```python
from build123d import *

# Parameters (mm, degrees)
F0_R     = 3.9243
F1_DEPTH = 2.54
F2_R     = 3.4925
F3_DEPTH = 25.4
F4_W     = 2.531840682
F4_H     = 6.5099929156
F5_DEPTH = 10.16
F6_R     = 1.524
F7_DEPTH = 25.4
F8_R     = 1.14299


# Not quite as in the source:
# - a fillet or chamfer is up to 0.001 mm smaller than in the source, because OpenCascade refuses the exact size


with BuildPart() as f1:
    # F0 (on Right) → F1 (new body)
    with BuildSketch(Plane.YZ):
        Circle(F0_R)
    extrude(amount=F1_DEPTH)

    # F2 (on face) → F3 (join)
    with BuildSketch(Plane.YZ.offset(2.54)):
        Circle(F2_R)
    extrude(amount=F3_DEPTH)

    # F4 (on face) → F5 (join)
    with BuildSketch(Plane.YZ.offset(27.94)):
        Rectangle(F4_W, F4_H)
    extrude(amount=F5_DEPTH)

    # F6 (on face) → F7 (cut)
    with BuildSketch(Plane(origin=(0, 1.265920341, 0), x_dir=(-1, 0, 0), z_dir=(0, 1, 0))):
        with Locations((-33.02, 0)):
            Circle(F6_R)
    extrude(amount=-F7_DEPTH, mode=Mode.SUBTRACT)

    # F8 (radius 1.143 in the source; OpenCascade refuses exactly that, so slightly less here)
    f8_edges = [f1.edges().sort_by_distance(p)[0] for p in [
        (38.1, 1.26592, 0),
        (38.1, -1.26592, 0),
        (33.02, 1.26592, 3.254996),
        (33.02, -1.26592, 3.254996),
        (33.02, 1.26592, -3.254996),
        (33.02, -1.26592, -3.254996),
    ]]
    fillet(f8_edges, radius=F8_R)


solid = f1.part
```
The model under review builds one solid part; all positions refer to its coordinate system, in mm. A direction names the side the tool comes from. Round coordinates to 2 decimals unless told otherwise and drop trailing zeros. Loops run counter-clockwise (first coordinate to the right, second up) from the corner with the lowest first, then second, coordinate; pieces in that order, holes last.
1) Consider section D-D on x = 6.5. State the section outline as (y, z) points (1 decimal), then the cut area to 3 significant figures.
Values follow:
outline: circle Ø7 at (0, 0)
area: 38.3 mm2
2) Wall thickness on line 1 along Z through (x, y) = (33.02, 0.25); line 2 along X through (y, z) = (2.75, -2.5); line 3 along X through (y, z) = (0.75, -1): over which ranges is each line inside the solid? List them lowest first.
Values follow:
line 1: z = -3.25 to -1.52, 1.52 to 3.25
line 2: x = 0 to 2.54
line 3: x = 0 to 31.87, 34.17 to 37.91
3) Tool access review of faces 5 (the face through (15.062, -0.455, 3.463)), 6 (the face through (33.09, 0.94, 2.91)), 7 (the face through (31, -1.266, 0)), 8 (the face through (31, 1.266, 0)), 9 (the face through (33.09, -0.92, -2.93)): name each direction out of +Z, -Z, +X, -X, +Y, -Y from which nothing blocks a thin tool from reaching the whole face with its end or side.
Values follow:
face 5: +X
face 6: +Z, +X, +Y
face 7: +Z, -Z, +X, -Y
face 8: +Z, -Z, +X, +Y
face 9: -Z, +X, -Y
4) Consider section B-B on z = 0. State the section outline as (x, y) points, then the cut area to 3 significant figures.
Values follow:
outline: (0, -3.92) - (2.54, -3.92) - (2.54, -3.49) - (27.94, -3.49) - (27.94, -1.27) - (31.5, -1.27) - (31.5, 1.27) - (27.94, 1.27) - (27.94, 3.49) - (2.54, 3.49) - (2.54, 3.92) - (0, 3.92) - close; (34.54, -1.27) - (36.96, -1.27) arc R1.14 ccw to (38.1, -0.12) - (38.1, 0.12) arc R1.14 ccw to (36.96, 1.27) - (34.54, 1.27) - close
area: 215 mm2
5) Consider section C-C on y = -2.75. State the section outline as (x, z) points, then the cut area to 3 significant figures.
Values follow:
outline: (0, -2.8) - (2.54, -2.8) - (2.54, -2.15) - (27.94, -2.15) - (27.94, 2.15) - (2.54, 2.15) - (2.54, 2.8) - (0, 2.8) - close
area: 124 mm2
6) The part is to be moulded in two halves that separate along X. For faces 1 (the face through (37.756, -0.94, 0.046)), 2 (the face through (34.543, 0.018, 0.067)), 3 (the face through (0, 0, 0)), 4 (the face through (33.09, -0.94, 2.91)), say which applies: pulls with the +X half, pulls with the -X half, needs draft (parallel to the pull), parting line crosses it, or undercut.
Values follow:
face 1: pulls with the +X half
face 2: undercut
face 3: pulls with the -X half
face 4: needs draft
7) Consider section A-A on x = 33.02. State the section outline as (y, z) points (3 decimals), then the cut area to 3 significant figures.
Values follow:
outline: (-1.266, -2.112) arc R1.143 ccw to (-0.123, -3.255) - (0.123, -3.255) arc R1.143 ccw to (1.266, -2.112) - (1.266, -1.524) - (-1.266, -1.524) - close; (-1.266, 1.524) - (1.266, 1.524) - (1.266, 2.112) arc R1.143 ccw to (0.123, 3.255) - (-0.123, 3.255) arc R1.143 ccw to (-1.266, 2.112) - close
area: 7.64 mm2
8) Clearance check with flat-ended pins moving along their axes: P1, Ø3.5, axis at x = 33.02, z = 0, coming from the +Y side; P2, Ø3, axis at x = 5, y = 2, coming from the +Z side; P3, Ø3.5, axis at x = 30.5, z = -0.5, coming from the -Y side. State where each tip first meets the part, or that it passes through.
Values follow:
P1: stops at y = 1.27
P2: stops at z = 3.46
P3: stops at y = -1.27
